For this review, take the finished solid that the model builds, in its own axes (mm). Face numbers are marked on the shaded views. Coordinates: 2 decimals unless noted, no trailing zeros. Loops run counter-clockwise (first coordinate to the right, second up) from the corner with the lowest first, then second, coordinate; pieces in that order, holes last. Notation, with made-up numbers: (-28, 78.5) -> (14, 78.5) arc R28 cw to (14, 104.5) -> close; hole circle Ø11 at (48, 87.5). An arc over 180 degrees is marked (long way). Use a Markdown table: item, result.
from build123d import *

# Parameters (mm, degrees)
F0_W     = 19.05
F0_H     = 101.6
F1_DEPTH = 6.35
F2_R     = 7.9375
F3_DEPTH = 25.4
F4_R     = 5.08


with BuildPart() as f1:
    # F0 (on Top) → F1 (new body)
    with BuildSketch(Plane.XY):
        with Locations((3.175, -6.782324)):
            Rectangle(F0_W, F0_H)
    extrude(amount=F1_DEPTH)

    # F2 (on face) → F3 (cut)
    with BuildSketch(Plane.XY.offset(6.35)):
        with Locations((3.175, 33.857676)):
            Circle(F2_R)
        with BuildLine():
            ThreePointArc((4.445, -51.232324), (2.276975, -50.334298), (3.175, -52.502324))
            ThreePointArc((3.175, -52.502324), (4.073026, -52.13035), (4.445, -51.232324))
        make_face()
    extrude(amount=-F3_DEPTH, mode=Mode.SUBTRACT)

    # F4
    f4_edges = [f1.edges().sort_by_distance(p)[0] for p in [
        (-6.35, 44.017676, 3.175),
        (-6.35, -57.582324, 3.175),
        (12.7, -57.582324, 3.175),
        (12.7, 44.017676, 3.175),
    ]]
    fillet(f4_edges, radius=F4_R)


solid = f1.part
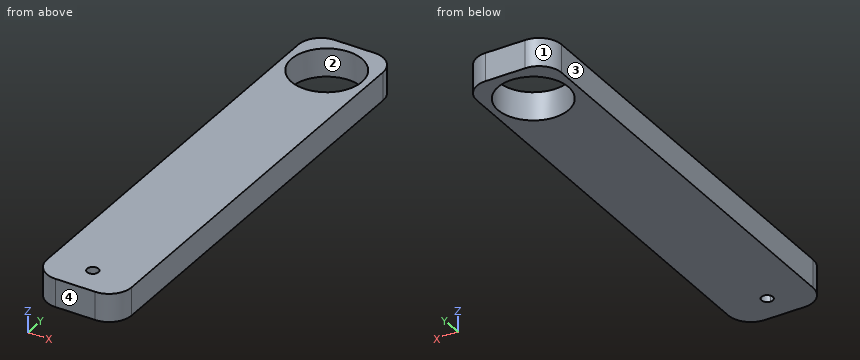
(1) Mouldability with a two-part tool opening along Y and no side actions: class the marked faces 1, 2, 3 and 4 as pulls with the +Y half, pulls with the -Y half, needs draft (parallel to the pull), parting line crosses it, or undercut.
Found:
| item | result |
|---|---|
| face 1 | pulls with the +Y half |
| face 2 | undercut |
| face 3 | needs draft |
| face 4 | pulls with the -Y half |
(2) For line 1 along Y through (x, z) = (2.5, 2.5); line 2 along Y through (x, z) = (9.5, 2.5); line 3 along Y through (x, z) = (9, 5.5), list the stretches that pass through material, from the lowest coordinate up.
Found:
| item | result |
|---|---|
| line 1 | y = -57.58 to -52.31, -50.16 to 25.95, 41.77 to 44.02 |
| line 2 | y = -57.22 to 29.06, 38.65 to 43.66 |
| line 3 | y = -57.39 to 28.47, 39.25 to 43.83 |
(3) Take a section at B-B on z = 2.5. State how many separate pieces and enclosed holes the cut face has, plus the area to 3 significant figures.
Found:
| item | result |
|---|---|
| separate pieces | 1 |
| enclosed holes | 2 |
| area | 1,710 mm^2 |
(4) For pin 1 Ø2 at (x, y) = (4.5, -10) entering from -Z, flat-tipped, find the tip position at first contact; note if it passes through.
Found:
| item | result |
|---|---|
| pin 1 | stops at z = 0 |
(5) Take a section at A-A on x = 0.75. Write out the cut boundary in (y, z), plus the area to 3 significant figures.
Found:
| item | result |
|---|---|
| outline | (-57.58, 0) -> (26.3, 0) -> (26.3, 6.35) -> (-57.58, 6.35) -> close; (41.42, 0) -> (44.02, 0) -> (44.02, 6.35) -> (41.42, 6.35) -> close |
| area | 549 mm^2 |
